Geometry check sheet. Reference: the model listing, model coordinates, mm. Face numbers are marked on the shaded views. Coordinates: 2 decimals unless noted, no trailing zeros. Loops run counter-clockwise (first coordinate to the right, second up) from the corner with the lowest first, then second, coordinate; pieces in that order, holes last. Notation, with made-up numbers: (83.25, 18.5) - (114.25, 18.5) arc R19 cw to (114.25, 45.5) - close; hole circle Ø4 at (44, -29). An arc over 180 degrees is marked (long way). One line per item, written item: value.
from build123d import *

# Parameters (mm, degrees)
SKETCH1_R           = 14.605
BOSS_EXTRUDE1_DEPTH = 1.5875
SKETCH3_R           = 28.575
BOSS_EXTRUDE2_DEPTH = 28.575
SKETCH4_R           = 17.4625
BOSS_EXTRUDE3_DEPTH = 43.815
CUT_EXTRUDE1_DEPTH  = 54.61


with BuildPart() as part:
    # Sketch1 → Revolve1 (revolve)
    with BuildSketch(Plane(origin=(0, 0, 0), x_dir=(0, 0, -1), z_dir=(1, 0, 0))):
        with Locations((0, 137.795)):
            Circle(SKETCH1_R)
    revolve(axis=Axis((0, 0, -1.447577339), (0, 0, 1)))

    # Sketch2 → Boss-Extrude1 (add, symmetric)
    with BuildSketch(Plane.XY):
        with BuildLine():
            Line((-128.390891494, 55.062409877), (-40.573034005, -4.124601434))
            ThreePointArc((-40.573034005, -4.124601434), (-28.871121899, -16.66875), (-23.858526625, -33.07497744))
            Line((-23.858526625, -33.07497744), (-16.51, -138.720978587))
            Line((-16.51, -138.720978587), (16.51, -138.720978587))
            Line((16.51, -138.720978587), (23.858526625, -33.07497744))
            ThreePointArc((23.858526625, -33.07497744), (28.871121899, -16.66875), (40.573034005, -4.124601434))
            Line((40.573034005, -4.124601434), (128.390891494, 55.062409877))
            Line((128.390891494, 55.062409877), (111.880891494, 83.65856871))
            Line((111.880891494, 83.65856871), (16.71450738, 37.199578874))
            ThreePointArc((16.71450738, 37.199578874), (0, 33.3375), (-16.71450738, 37.199578874))
            Line((-16.71450738, 37.199578874), (-111.880891494, 83.65856871))
            Line((-111.880891494, 83.65856871), (-128.390891494, 55.062409877))
        make_face()
    extrude(amount=BOSS_EXTRUDE1_DEPTH, both=True)

    # Sketch3 → Boss-Extrude2 (add)
    with BuildSketch(Plane(origin=(0, 0, -1.5875), x_dir=(-1, 0, 0), z_dir=(0, 0, -1))):
        Circle(SKETCH3_R)
    extrude(amount=BOSS_EXTRUDE2_DEPTH)

    # Sketch4 → Boss-Extrude3 (add)
    with BuildSketch(Plane(origin=(0, 0, -30.1625), x_dir=(-1, 0, 0), z_dir=(0, 0, -1))):
        Circle(SKETCH4_R)
    extrude(amount=BOSS_EXTRUDE3_DEPTH)

    # Sketch6 → Cut-Extrude1 (cut)
    with BuildSketch(Plane(origin=(0, 0, -73.9775), x_dir=(-1, 0, 0), z_dir=(0, 0, -1))):
        Polygon((12.7, -7.332348419), (12.7, 7.332348419), (0, 14.664696837), (-12.7, 7.332348419), (-12.7, -7.332348419), (0, -14.664696837), align=None)
    extrude(amount=-CUT_EXTRUDE1_DEPTH, mode=Mode.SUBTRACT)


solid = part.part
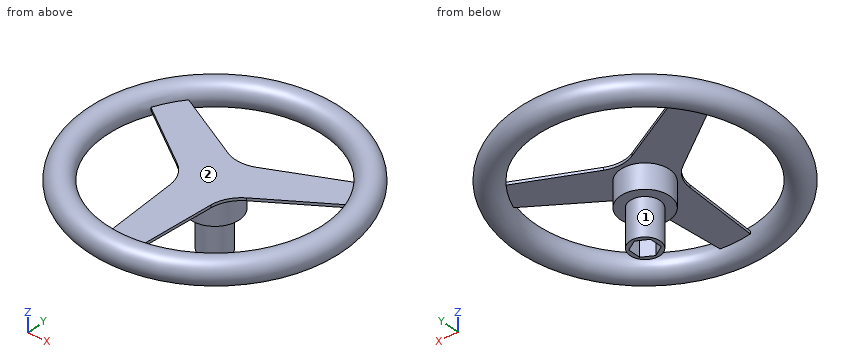
(1) Cross-section at C-C on x = 76.5. State how many separate pieces and enclosed holes the cut face has, and give its area (3 significant figures).
Reply:
separate pieces: 3
enclosed holes: 0
area: 1,760 mm2
(2) Release check for a two-part mould opening along X. For the marked faces 1 and 2 record: pulls with the +X half, pulls with the -X half, needs draft (parallel to the pull), parting line crosses it, or undercut.
Reply:
face 1: parting line crosses it
face 2: undercut
(3) Go/stop test with flat-tipped pins: pin 1 Ø7.5 at (y, z) = (1, -46) entering from +X; pin 2 Ø4 at (x, y) = (69, 54) entering from +Z; pin 3 Ø2 at (y, z) = (-11, -2.5) entering from +X. Record where each tip stops, or that it passes through.
Reply:
pin 1: x = 17.46
pin 2: z = 1.59
pin 3: x = 151.95
(4) Material ranges on probe 1 along Y at (x, z) = (20.5, -3); probe 2 along X at (y, z) = (16.5, -12); probe 3 along Z at (x, y) = (2, -27), recorded low to high. Write a range as from..to.
Reply:
probe 1: -150.7..-121.79, -19.91..19.91, 121.79..150.7
probe 2: -145.19..-128.41, -23.33..23.33, 128.41..145.19
probe 3: -30.16..1.59
(5) Cross-section at B-B on y = 0. Record the cut outline in (x, z) (1 decimal).
Reply:
outline: circle Ø29.2 at (-137.8, 0); (-46.7, -1.6) - (-28.6, -1.6) - (-28.6, -30.2) - (-17.5, -30.2) - (-17.5, -74) - (-12.7, -74) - (-12.7, -19.4) - (12.7, -19.4) - (12.7, -74) - (17.5, -74) - (17.5, -30.2) - (28.6, -30.2) - (28.6, -1.6) - (46.7, -1.6) - (46.7, 1.6) - (-46.7, 1.6) - close; circle Ø29.2 at (137.8, 0)
(6) Cross-section at A-A on z = -61. Record the cut outline in (x, y) (1 decimal).
Reply:
outline: circle Ø34.9 at (0, 0); hole (-12.7, -7.3) - (0, -14.7) - (12.7, -7.3) - (12.7, 7.3) - (0, 14.7) - (-12.7, 7.3) - close
